from build123d import *

# Parameters (mm, degrees)
F0_R     = 14.4907
F0_R_2   = 7.9883
F1_DEPTH = 6.35
F2_R     = 14.4907
F2_R_2   = 7.9883
F3_DEPTH = 8.382
F4_R     = 1.5875
F5_DEPTH = 15.1638
F6_R     = 1.5875
F7_DEPTH = 15.4178


with BuildPart() as f1:
    # F0 (on Front) → F1 (new body)
    with BuildSketch(Plane.XZ):
        Circle(F0_R)
        Circle(F0_R_2, mode=Mode.SUBTRACT)
    extrude(amount=F1_DEPTH)

    # F2 (on face) → F3 (join)
    with BuildSketch(Plane.XZ.offset(6.35)):
        Circle(F2_R)
        Circle(F2_R_2, mode=Mode.SUBTRACT)
    extrude(amount=F3_DEPTH)

    # F4 (on Right) → F5 (cut, symmetric)
    with BuildSketch(Plane.YZ):
        with Locations((-3.175, 0)):
            Circle(F4_R)
    extrude(amount=F5_DEPTH, both=True, mode=Mode.SUBTRACT)

    # F6 (on Top) → F7 (cut, symmetric)
    with BuildSketch(Plane.XY):
        with Locations((0, -3.175)):
            Circle(F6_R)
    extrude(amount=F7_DEPTH, both=True, mode=Mode.SUBTRACT)

    # F9: sweep along a path in F0
    with BuildLine(Plane.XZ) as f9_path:
        CenterArc((0, 0), 14.4907, 0, 360)
    # F8 (on Right) → F9 (sweep, cut)
    with BuildSketch(Plane.YZ):
        Polygon((0, 14.501917), (0, 16.049927), (-6.35176, 16.049927), (-6.35176, 14.501917), (-3.17588, 13.768708), align=None)
    sweep(path=f9_path.line, mode=Mode.SUBTRACT)


solid = f1.part
Here's how the part is built. I have some questions about the finished solid (model axes, mm). A direction names the side the tool comes from. Coordinates: 2 decimals unless noted, no trailing zeros. Write each loop counter-clockwise with the first axis right and the second up, starting at its lowest first coordinate (ties: lowest second). Pieces come first, ordered by that corner, then holes.
1) If we section it at D-D (y = -9.75): List the corners of the cut face in (x, z) for me, plus the area to 3 significant figures.
Filled in:
outline: circle Ø28.98 at (0, 0); hole circle Ø15.98 at (0, 0)
area: 459 mm2
2) If I drill on line 1 (Y direction, x = 11.25, z = 0); line 2 (Z direction, x = -7.25, y = -11.25); line 3 (Z direction, x = 0, y = -10.75), over which ranges is the centre line in solid material (lowest first)?
Filled in:
line 1: y = -14.73 to -4.76, -1.59 to 0
line 2: z = -12.55 to -3.35, 3.35 to 12.55
line 3: z = -14.49 to -7.99, 7.99 to 14.49
3) Thinking about a two-plate mould opening in Y: for faces 1 (the face through (6, -14.732, -6)), 2 (the face through (11.03, -1.66, 0.48)), 3 (the face through (1.466, -3.783, -10.936)), 4 (the face through (6, 0, -6)), which applies, +Y half, -Y half, draft (parallel to the pull), parting line (faces both ways), or undercut?
Filled in:
face 1: -Y half
face 2: undercut
face 3: undercut
face 4: +Y half
4) If we section it at B-B (y = -2.25): List the corners of the cut face in (x, z) for me, plus the area to 3 significant figures.
Filled in:
outline: (-13.92, -1.29) arc R13.98 ccw to (-1.29, -13.92) - (-1.29, -7.88) arc R7.99 cw to (-7.88, -1.29) - close; (-13.92, 1.29) - (-7.88, 1.29) arc R7.99 cw to (-1.29, 7.88) - (-1.29, 13.92) arc R13.98 ccw to start; (1.29, -13.92) arc R13.98 ccw to (13.92, -1.29) - (7.88, -1.29) arc R7.99 cw to (1.29, -7.88) - close; (1.29, 7.88) arc R7.99 cw to (7.88, 1.29) - (13.92, 1.29) arc R13.98 ccw to (1.29, 13.92) - close
area: 352 mm2
5) I'm going to push flat-ended pins straight in: pin 1 (1.5 mm diameter, centred on x = -7.5, y = -5.5, fed in from -Z); pin 2 (1 mm diameter, centred on y = -2, z = 10.5, fed in from -X); pin 3 (2 mm diameter, centred on x = -2.5, y = -3.5, fed in from +Z). Where does each tip first touch, or does it pass through?
Filled in:
pin 1: stops at z = -12.66
pin 2: stops at x = -9.88
pin 3: stops at z = 13.9
6) Which directions (+Z, -Z, +X, -X, +Y, -Y) give clear straight access to the entire face, cutting with the end or side of a thin tool? Please do faces 5 (the face through (-10.938, -2.442, -1.408)), 6 (the face through (12.76, -2.98, -5.29)).
Filled in:
face 5: +X, -X
face 6: none
7) If we section it at A-A (x = 0): Count the separate pieces of the cut face and the enclosed holes in it, plus the area to 3 significant figures.
Filled in:
separate pieces: 4
enclosed holes: 0
area: 149 mm2
